from build123d import *

# Parameters (mm, degrees)
BOSS_EXTRUDE1_DEPTH = 3.5
SKETCH2_R           = 0.8
SCREW_HOLES_DEPTH   = 37.028935124
SKETCH3_W           = 4
SKETCH3_H           = 14
BOSS_EXTRUDE2_DEPTH = 8
CUT_EXTRUDE1_DEPTH  = 1.5
CUT_EXTRUDE2_START  = 13
SKETCH5_R           = 0.8
CUT_EXTRUDE2_DEPTH  = 50.74008936
FILLET1_R           = 3.5


with BuildPart() as part:
    # Sketch1 → Boss-Extrude1 (new body)
    with BuildSketch(Plane(origin=(0, 0, 0), x_dir=(1, 0, 0), z_dir=(0, 1, 0))):
        with BuildLine():
            Line((17, -10), (17, -12.105263158))
            Line((17, -12.105263158), (26, -11.631578947))
            Line((26, -11.631578947), (26, 0))
            ThreePointArc((26, 0), (28.126845638, 6.820617489), (33.753470489, 11.223501553))
            Line((33.753470489, 11.223501553), (17, 12.105263158))
            Line((17, 12.105263158), (17, 10))
            Line((17, 10), (17, 7))
            Line((17, 7), (13, 7))
            Line((13, 7), (13, 0))
            Line((13, 0), (13, -7))
            Line((13, -7), (17, -7))
            Line((17, -7), (17, -10))
        make_face()
    extrude(amount=-BOSS_EXTRUDE1_DEPTH)

    # Sketch2 → Screw Holes (cut, through all)
    with BuildSketch(Plane(origin=(0, 0, 0), x_dir=(1, 0, 0), z_dir=(0, 1, 0))):
        with Locations(Location((24, 8.5, 0), (0, 0, 270))):
            Circle(SKETCH2_R)
        with Locations(Location((24, -8.5, 0), (0, 0, 270))):
            Circle(SKETCH2_R)
    extrude(amount=-SCREW_HOLES_DEPTH, mode=Mode.SUBTRACT)

    # Sketch3 → Boss-Extrude2 (add)
    with BuildSketch(Plane(origin=(0, 0, 0), x_dir=(1, 0, 0), z_dir=(0, 1, 0))):
        with Locations((15, 0)):
            Rectangle(SKETCH3_W, SKETCH3_H)
    extrude(amount=-BOSS_EXTRUDE2_DEPTH)

    # Sketch4 → Cut-Extrude1 (cut)
    with BuildSketch(Plane(origin=(0, 0, 0), x_dir=(1, 0, 0), z_dir=(0, 1, 0))):
        Polygon((13, 0), (13, 3), (26.381049961, 3), (26.381049961, -3), (13, -3), align=None)
    extrude(amount=-CUT_EXTRUDE1_DEPTH, mode=Mode.SUBTRACT)

    # Sketch5 → Cut-Extrude2 (cut, through all)
    with BuildSketch(Plane.XY.offset(CUT_EXTRUDE2_START)):
        with Locations((15, -6)):
            Circle(SKETCH5_R)
    extrude(amount=-CUT_EXTRUDE2_DEPTH, mode=Mode.SUBTRACT)

    # Fillet1
    # the kernel refuses this fillet: 3.5 mm, written as the material it takes off along each edge
    with BuildSketch(Plane(origin=(8.262093993, -3.5, 12.565152948), x_dir=(0, 1, 0), z_dir=(0.9986178293325098, 0, -0.05255883312276359))) as fillet1_piece_1_section:
        with BuildLine():
            CenterArc((FILLET1_R, -FILLET1_R), FILLET1_R, 90, 90)
            Line((0, -FILLET1_R), (-FILLET1_R * 0.02, -FILLET1_R))
            Line((-FILLET1_R * 0.02, -FILLET1_R), (-FILLET1_R * 0.02, FILLET1_R * 0.02))
            Line((-FILLET1_R * 0.02, FILLET1_R * 0.02), (FILLET1_R, FILLET1_R * 0.02))
            Line((FILLET1_R, FILLET1_R * 0.02), (FILLET1_R, 0))
        make_face()
    fillet1_piece_1 = extrude(amount=26.512456753, mode=Mode.PRIVATE)
    fillet1_piece_1 = split(fillet1_piece_1, bisect_by=Plane(origin=(17, -2.7076171, 11.074941428), z_dir=(1, 0, 0)), keep=Keep.TOP, mode=Mode.PRIVATE)
    fillet1_piece_1 = split(fillet1_piece_1, bisect_by=Plane(origin=(26, -2.7076171, 11.074941428), z_dir=(-1, 0, 0)), keep=Keep.TOP, mode=Mode.PRIVATE)
    add(fillet1_piece_1, mode=Mode.SUBTRACT)
    with BuildSketch(Plane(origin=(42.491376496, -3.5, -10.763611763), x_dir=(-0.05255883312276374, 0, 0.9986178293325098), z_dir=(-0.9986178293325098, 0, -0.05255883312276374))) as fillet1_piece_2_section:
        with BuildLine():
            CenterArc((FILLET1_R, FILLET1_R), FILLET1_R, 180, 90)
            Line((0, FILLET1_R), (-FILLET1_R * 0.02, FILLET1_R))
            Line((-FILLET1_R * 0.02, FILLET1_R), (-FILLET1_R * 0.02, -FILLET1_R * 0.02))
            Line((-FILLET1_R * 0.02, -FILLET1_R * 0.02), (FILLET1_R, -FILLET1_R * 0.02))
            Line((FILLET1_R, -FILLET1_R * 0.02), (FILLET1_R, 0))
        make_face()
    fillet1_piece_2 = extrude(amount=34.276658695, mode=Mode.PRIVATE)
    fillet1_piece_2 = split(fillet1_piece_2, bisect_by=Plane(origin=(17, -2.672351217, -10.961883327), z_dir=(1, 0, 0)), keep=Keep.TOP, mode=Mode.PRIVATE)
    fillet1_piece_2 = fillet1_piece_2 - Plane(origin=(38, -2.672351217, 0), x_dir=(-1, 0, 0), z_dir=(0, 1, 0)) * Cylinder(12, 83, mode=Mode.PRIVATE)
    add(fillet1_piece_2, mode=Mode.SUBTRACT)


solid = part.part
Verification items for the finished model (mm, model axes). A direction names the side the tool comes from. Coordinates: 2 decimals unless noted, no trailing zeros. Order: outer loops, then holes, each group sorted by start corner. A loop starts at its lowest first (then second) coordinate and runs counter-clockwise, first axis right, second up. Notation, with made-up numbers: M 13,-6.75 L 38,-6.75 A33 ccw 38,25.25 Z; hole C 58,28 d11. An arc over 180 degrees is marked long. One line per item, written item: value. Start each with the question number.
Item 1: Mould release check, pull along X, two halves, no side actions. Record for faces 1 (the flat face through (21, 0, 7)), 2 (the cylindrical face through (14.37, -6.49, 0.1)), 3 (the cylindrical face through (21.48, -2.45, 10.87)): pulls with the +X half, pulls with the -X half, needs draft (parallel to the pull), parting line crosses it, or undercut.
Item 2: Sectioned sample at B-B on x = 15. Record the cut outline in (y, z).
Item 3: Thickness scan on probe 1 along Y at (x, z) = (15, 0.5); probe 2 along X at (y, z) = (-1.95, 8.5); probe 3 along Y at (x, z) = (19, 2). Record the ranges inside material, lowest first.
Item 4: Access from +Z, -Z, +X, -X, +Y, -Y to the whole of each face (thin tool, end or side, straight path). Record for faces 4 (the flat face through (20, -1.5, 0)), 5 (the flat face through (26, -2, 6)), 6 (the flat face through (17, -2, 10)), 7 (the flat face through (17, -2, -9)).
Item 5: Depth check by flat-ended pin: P1, Ø1.8, axis at y = -1, z = 8, coming from the +X side; P2, Ø1.5, axis at x = 25.5, y = -5.5, coming from the +Z side (3 decimals); P3, Ø4.5, axis at x = 14, y = -5, coming from the -Z side; P4, Ø2, axis at x = 30.5, y = -4, coming from the -Z side. Enter the tip coordinate at first touch or a pass-through.
Item 6: Sectioned sample at D-D on y = -3. Record the cut outline in (x, z), then the cut area to 3 significant figures.
Item 7: Sectioned sample at A-A on y = -6. Record the cut outline in (x, z).
Item 8: Sectioned sample at C-C on z = -3.5. Record the cut outline in (x, y).
Calculated:
1. face 1: needs draft
1. face 2: undercut
1. face 3: pulls with the +X half
2. outline: M -8,-7 L -6.8,-7 L -6.8,7 L -8,7 Z; M -5.2,-7 L 0,-7 L 0,-3 L -1.5,-3 L -1.5,3 L 0,3 L 0,7 L -5.2,7 Z
3. probe 1: -8 to -6.8, -5.2 to -1.5
3. probe 2: 17 to 23.2, 24.8 to 26
3. probe 3: -3.5 to -1.5
4. face 4: +X, -X, +Y
4. face 5: +Z, +X, +Y, -Y
4. face 6: +Z, -X, +Y, -Y
4. face 7: -Z, -X, +Y, -Y
5. P1: x = 26
5. P2: through
5. P3: z = -7
5. P4: z = -9.7
6. outline: M 13,-7 L 17,-7 L 17,-10.41 L 30.9,-9.67 A12 cw 26,0 L 26,9.93 L 17,10.41 L 17,7 L 13,7 Z; hole C 24,-8.5 d1.6; hole C 24,8.5 d1.6
6. area: 250 mm^2
7. outline: M 13,-7 L 14.2,-7 L 14.2,7 L 13,7 Z; M 15.8,-7 L 17,-7 L 17,7 L 15.8,7 Z
8. outline: M 13,-8 L 17,-8 L 17,-3.5 L 26.52,-3.5 L 26.52,0 L 13,0 Z; hole C 15,-6 d1.6
